Source: three-view drawing plus pictorial views. Frame: mm from the lowest corner of the part. A direction names the side the tool comes from. Give positions to 0.01 mm unless a question says otherwise; leave off trailing zeros. Write each loop counter-clockwise with the first axis right and the second up, starting at its lowest first coordinate (ties: lowest second). Pieces come first, ordered by that corner, then holes.
Q1. Line query: L1, parallel to X at y = 5, z = 7 (1 decimal); L2, parallel to Y at x = 6, z = 3.25 (1 decimal); L3, parallel to Y at x = 8.5, z = 7.25 (1 decimal). Output: solid intervals per line, ascending.
Q2. Cut plane B-B on y = 3.5. Return the cut outline in (x, z).
Q3. Cut plane A-A on z = 3.5. Return the cut outline in (x, y).
Q4. Cut plane C-C on x = 7. Return the cut outline in (y, z).
Q5. Pin query (flat end, axial travel): pin 1 (1.5 mm diameter, centred on x = 9.5, y = 8.5, fed in from +Z); pin 2 (2 mm diameter, centred on y = 7, z = 3.5, fed in from +X); pin 3 (3 mm diameter, centred on y = 8, z = 2, fed in from -X). Return the tip coordinate at first contact, or that it passes through.
Q6. Draft query along X for the marked faces 1, 2 and 3. Return one class per face: pulls with the +X half, pulls with the -X half, needs draft (parallel to the pull), parting line crosses it, or undercut.
Q7. Cut plane D-D on y = 8. Return the cut outline in (x, z) (1 decimal), plus the area to 3 significant figures.
Q8. Reachability of the marked faces 4 and 5 from +Z, -Z, +X, -X, +Y, -Y: full face, straight path, thin tool, end or side. Return the list, or none.
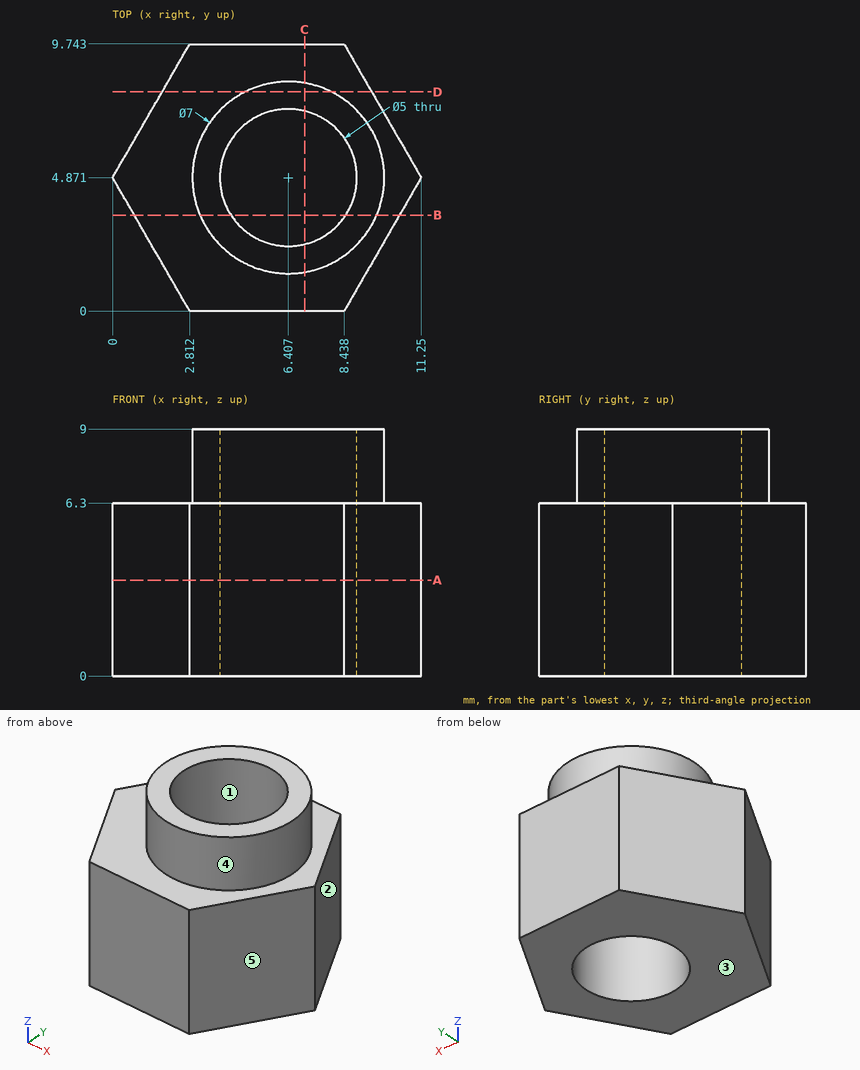
Data:
1. L1: x = 2.9 to 3.9, 8.9 to 9.9
1. L2: y = 0 to 2.4, 7.3 to 9.7
1. L3: y = 2.1 to 3.5, 6.2 to 7.7
2. outline: (0.79, 0) - (4.32, 0) - (4.32, 9) - (3.19, 9) - (3.19, 6.3) - (0.79, 6.3) - close; (8.5, 0) - (10.46, 0) - (10.46, 6.3) - (9.63, 6.3) - (9.63, 9) - (8.5, 9) - close
3. outline: (0, 4.87) - (2.81, 0) - (8.44, 0) - (11.25, 4.87) - (8.44, 9.74) - (2.81, 9.74) - close; hole circle Ø5 at (6.41, 4.87)
4. outline: (0, 0) - (2.44, 0) - (2.44, 9) - (1.42, 9) - (1.42, 6.3) - (0, 6.3) - close; (7.3, 0) - (9.74, 0) - (9.74, 6.3) - (8.32, 6.3) - (8.32, 9) - (7.3, 9) - close
5. pin 1: stops at z = 6.3
5. pin 2: stops at x = 10.6
5. pin 3: stops at x = 0.94
6. face 1: undercut
6. face 2: pulls with the +X half
6. face 3: needs draft
7. outline: (1.8, 0) - (9.4, 0) - (9.4, 6.3) - (8, 6.3) - (8, 9) - (4.8, 9) - (4.8, 6.3) - (1.8, 6.3) - close
7. area: 56.6 mm2
8. face 4: +Z
8. face 5: +Z, -Z, +X, -Y
